from build123d import *

# Parameters (mm, degrees)
BASE_EXTRUDE_DEPTH = 15
HOLE1_D            = 5
HOLE1_DEPTH        = 14
HOLE1_TIP          = 1.502151548


with BuildPart() as part:
    # Sketch1 → Base-Extrude (new body)
    with BuildSketch(Plane.XY):
        with BuildLine():
            Line((33.25, 44), (15.25, 44))
            ThreePointArc((15.25, 44), (13.128679656, 43.121320344), (12.25, 41))
            Line((12.25, 41), (12.25, 0))
            ThreePointArc((12.25, 0), (10.76763809, -1.931851653), (8.517949192, -1))
            ThreePointArc((8.517949192, -1), (7.785898385, -0.267949192), (6.785898385, 0))
            Line((6.785898385, 0), (-6.785898385, 0))
            ThreePointArc((-6.785898385, 0), (-7.785898385, -0.267949192), (-8.517949192, -1))
            ThreePointArc((-8.517949192, -1), (-10.76763809, -1.931851653), (-12.25, 0))
            Line((-12.25, 0), (-12.25, 41))
            ThreePointArc((-12.25, 41), (-13.128679656, 43.121320344), (-15.25, 44))
            Line((-15.25, 44), (-33.25, 44))
            ThreePointArc((-33.25, 44), (-35.371320344, 43.121320344), (-36.25, 41))
            Line((-36.25, 41), (-36.25, -21.226497308))
            ThreePointArc((-36.25, -21.226497308), (-34.910254038, -26.226497308), (-31.25, -29.886751346))
            Line((-31.25, -29.886751346), (-11.686313468, -41.181851032))
            ThreePointArc((-11.686313468, -41.181851032), (-10.930794046, -41.801889798), (-10.414674871, -42.631876946))
            Line((-10.414674871, -42.631876946), (0.982897316, -70.148050297))
            ThreePointArc((0.982897316, -70.148050297), (2.087825215, -71.494408837), (3.754535914, -72))
            Line((3.754535914, -72), (64.040943269, -72))
            ThreePointArc((64.040943269, -72), (66.571117606, -70.611898825), (66.75986663, -67.732145215))
            Line((66.75986663, -67.732145215), (42.229318474, -15.126214931))
            ThreePointArc((42.229318474, -15.126214931), (41.951097171, -13.989218308), (42.129163973, -12.832299716))
            Line((42.129163973, -12.832299716), (43.697595308, -8.52307004))
            ThreePointArc((43.697595308, -8.52307004), (43.87566211, -7.366151448), (43.597440806, -6.229154825))
            Line((43.597440806, -6.229154825), (37.18692213, 7.518246841))
            ThreePointArc((37.18692213, 7.518246841), (36.487039929, 9.580033319), (36.25, 11.744429459))
            Line((36.25, 11.744429459), (36.25, 41))
            ThreePointArc((36.25, 41), (35.371320344, 43.121320344), (33.25, 44))
        make_face()
    extrude(amount=-BASE_EXTRUDE_DEPTH)

    # Hole1
    with Locations(Plane(origin=(0, 44, 0), x_dir=(-1, 0, 0), z_dir=(0, 1, 0))):
        with Locations((22, -7.5), (-22, -7.5)):
            Hole(HOLE1_D / 2, depth=HOLE1_DEPTH)
            with Locations((0, 0, -(HOLE1_DEPTH + HOLE1_TIP / 2))):  # 118° drill point
                Cone(0, HOLE1_D / 2, HOLE1_TIP, mode=Mode.SUBTRACT)


solid = part.part
Could you check a few things on this model? Use its own coordinates, in mm. A direction names the side the tool comes from. Coordinates: 2 decimals unless noted, no trailing zeros. Order: outer loops, then holes, each group sorted by start corner. A loop starts at its lowest first (then second) coordinate and runs counter-clockwise, first axis right, second up. Notation, with made-up numbers: (-26, 27.25) - (18, 27.25) arc R7 cw to (18, 38.25) - close; hole circle Ø2 at (-6, -17). An arc over 180 degrees is marked (long way). Answer in a Markdown table with one row per item. Add a question column.
(1) Will these pins go through, and if not, where does the flat tip stop? pin 1 (2 mm diameter, centred on y = -57.5, z = -13, fed in from -X); pin 2 (3 mm diameter, centred on x = -22, z = -7.5, fed in from -Y); pin 3 (5 mm diameter, centred on y = 21, z = -3, fed in from +X).
(2) If we section it at B-B, the plane z = -13: Please give me the cut outline in (x, y).
(3) If we section it at C-C, the plane x = 39.5: Please give me the cut outline in (y, z).
(4) If we mould it in two halves opening along X, with no side actions, what happens to faces 4 (the face through (36.494, 9.55, -7.395)), 5 (the face through (-24.1, 44, -5.7)), 6 (the face through (-22.4, 28.76, -7.67))? For each: released by +X, released by -X, zero draft, split by the parting line, or undercut.
(5) If we section it at A-A, the plane y = 14.5: Please give me the cut outline in (x, z).
(6) I need wall thicknesses on L1, parallel to X at y = 38.5, z = -7.5; L2, parallel to Z at x = -22, y = 35; L3, parallel to X at y = 18.5, z = -7.75. Which ranges of each line are inside material? Lowest first, please.
(7) On a 3-axis mill with a long thin cutter (end or side, diameter ignored), from which of +Z, -Z, +X, -X, +Y, -Y can I reach the whole of each face in a straight line? I mean faces 1 (the face through (20, 37, -9)), 2 (the face through (42.9, -10.71, -7.4)), 3 (the face through (0, 0, -7)). Say none if no direction works.
(8) If we section it at D-D, the plane y = -3.5: Please give me the cut outline in (x, z).
Results are:
| question | item | result |
|---|---|---|
| 1 | pin 1 | stops at x = -4.67 |
| 1 | pin 2 | stops at y = -36.09 |
| 1 | pin 3 | stops at x = 36.25 |
| 2 | outline | (-36.25, -21.23) arc R10 ccw to (-31.25, -29.89) - (-11.69, -41.18) arc R3 cw to (-10.41, -42.63) - (0.98, -70.15) arc R3 ccw to (3.75, -72) - (64.04, -72) arc R3 ccw to (66.76, -67.73) - (42.23, -15.13) arc R3 cw to (42.13, -12.83) - (43.7, -8.52) arc R3 ccw to (43.6, -6.23) - (37.19, 7.52) arc R10 cw to (36.25, 11.74) - (36.25, 41) arc R3 ccw to (33.25, 44) - (15.25, 44) arc R3 ccw to (12.25, 41) - (12.25, 0) arc R2 cw to (8.52, -1) arc R2 ccw to (6.79, 0) - (-6.79, 0) arc R2 ccw to (-8.52, -1) arc R2 cw to (-12.25, 0) - (-12.25, 41) arc R3 ccw to (-15.25, 44) - (-33.25, 44) arc R3 ccw to (-36.25, 41) - close |
| 3 | outline | (-72, -15) - (2.56, -15) - (2.56, 0) - (-72, 0) - close |
| 4 | face 4 | released by +X |
| 4 | face 5 | zero draft |
| 4 | face 6 | undercut |
| 5 | outline | (-36.25, -15) - (-12.25, -15) - (-12.25, 0) - (-36.25, 0) - close; (12.25, -15) - (36.25, -15) - (36.25, 0) - (12.25, 0) - close |
| 6 | L1 | x = -36.25 to -24.5, -19.5 to -12.25, 12.25 to 19.5, 24.5 to 36.25 |
| 6 | L2 | z = -15 to -10, -5 to 0 |
| 6 | L3 | x = -36.25 to -12.25, 12.25 to 36.25 |
| 7 | face 1 | +Y |
| 7 | face 2 | +Z, -Z, +X |
| 7 | face 3 | +Z, -Z, +Y |
| 8 | outline | (-36.25, -15) - (42.32, -15) - (42.32, 0) - (-36.25, 0) - close |
